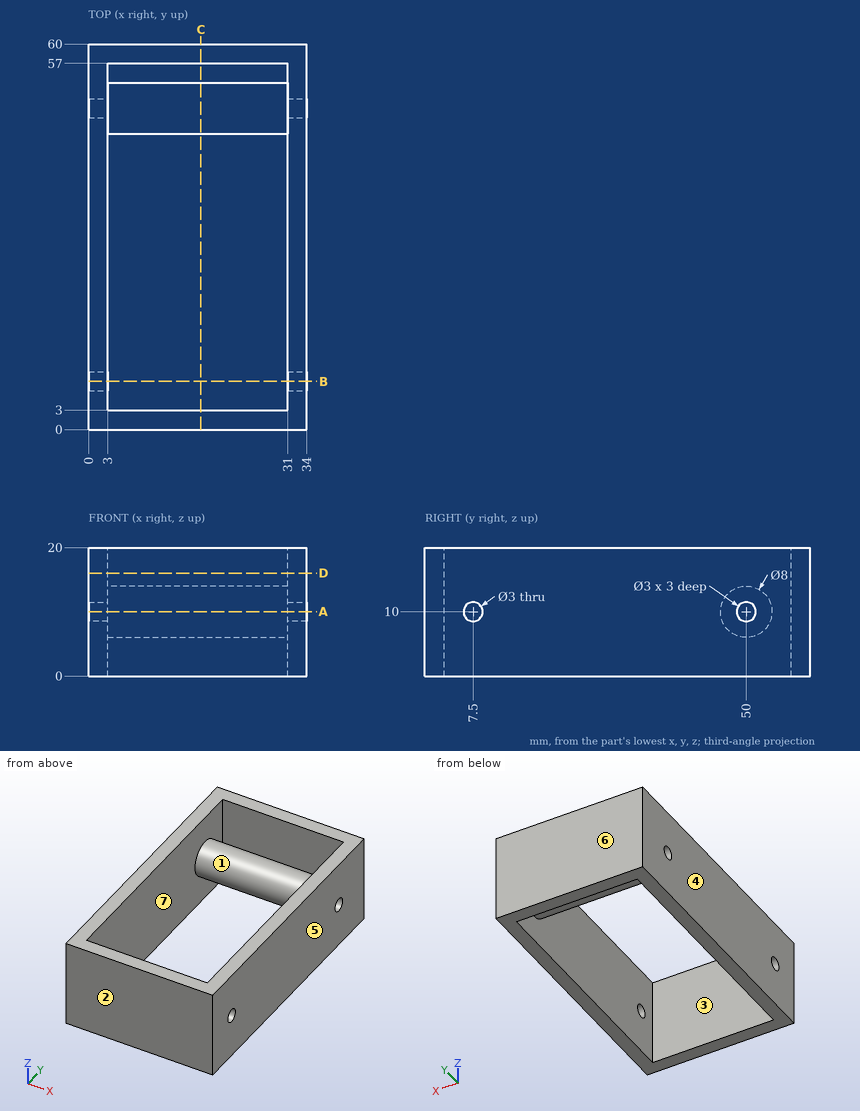
For this review, use the dimensioned drawing (mm, ordinates from the lowest corner) and the shaded views. A direction names the side the tool comes from. Round coordinates to 2 decimals unless told otherwise and drop trailing zeros. Write each loop counter-clockwise with the first axis right and the second up, starting at its lowest first coordinate (ties: lowest second). Pieces come first, ordered by that corner, then holes. Notation, with made-up numbers: M 50,72 L 70,72 A22 ccw 70,108 Z; hole C 2,-31 d1. An arc over 180 degrees is marked long. Answer as CSV lines item,"result". Start each with the question number.
Q1. Consider section C-C, the plane x = 17.5. Give the boundary of the cut face in (y, z).
Q2. Tool access review of the marked faces 1, 2 and 3: name each direction out of +Z, -Z, +X, -X, +Y, -Y from which nothing blocks a thin tool from reaching the whole face with its end or side.
Q3. Consider section B-B, the plane y = 7.5. Give the boundary of the cut face in (x, z), then the cut area to 3 significant figures.
Q4. Wall thickness on line 1 along Y through (x, z) = (32.1, 10); line 2 along X through (y, z) = (33, 16.75); line 3 along Y through (x, z) = (4.5, 3.5): over which ranges is each line inside the solid? List them lowest first.
Q5. Consider section D-D, the plane z = 16. Give the boundary of the cut face in (x, y), then the cut area to 3 significant figures.
Q6. Consider section A-A, the plane z = 10. Give the boundary of the cut face in (x, y).
Q7. The part is to be moulded in two halves that separate along X. For the marked faces 4, 5, 6 and 7, say which applies: +X half, -X half, draft (parallel to the pull), parting line (faces both ways), or undercut.
Q8. Clearance check with flat-ended pins moving along their axes: P1, Ø2.5, axis at y = 50, z = 10, coming from the -X side; P2, Ø2.5, axis at y = 50, z = 10, coming from the +X side. State where each tip first meets the part, or that it passes through.
Result set:
1,outline,"M 0,0 L 3,0 L 3,20 L 0,20 Z; C 50,10 d8; M 57,0 L 60,0 L 60,20 L 57,20 Z"
2,face 1,"none"
2,face 2,"+Z, -Z, +X, -X, -Y"
2,face 3,"+Z, -Z"
3,outline,"M 0,0 L 3,0 L 3,8.5 L 0,8.5 Z; M 0,11.5 L 3,11.5 L 3,20 L 0,20 Z; M 31,0 L 34,0 L 34,8.5 L 31,8.5 Z; M 31,11.5 L 34,11.5 L 34,20 L 31,20 Z"
3,area,"102 mm²"
4,line 1,"y = 0 to 6, 9 to 48.5, 51.5 to 60"
4,line 2,"x = 0 to 3, 31 to 34"
4,line 3,"y = 0 to 3, 57 to 60"
5,outline,"M 0,0 L 34,0 L 34,60 L 0,60 Z; hole M 3,3 L 31,3 L 31,57 L 3,57 Z"
5,area,"528 mm²"
6,outline,"M 0,0 L 34,0 L 34,6 L 31,6 L 31,3 L 3,3 L 3,6 L 0,6 Z; M 0,9 L 3,9 L 3,46 L 31,46 L 31,9 L 34,9 L 34,48.5 L 31,48.5 L 31,51.5 L 34,51.5 L 34,60 L 0,60 L 0,51.5 L 3,51.5 L 3,48.5 L 0,48.5 Z; hole M 3,54 L 31,54 L 31,57 L 3,57 Z"
7,face 4,"-X half"
7,face 5,"+X half"
7,face 6,"draft"
7,face 7,"undercut"
8,P1,"stops at x = 3"
8,P2,"stops at x = 31"
